Verification items for this drawing (mm, ordinates from the low corner). Coordinates: 2 decimals unless noted, no trailing zeros. Write each loop counter-clockwise with the first axis right and the second up, starting at its lowest first coordinate (ties: lowest second). Pieces come first, ordered by that corner, then holes. Notation, with made-up numbers: (46.5, -0.5) -> (56.5, -0.5) arc R28 ccw to (56.5, 35.5) -> close; hole circle Ø11 at (70.25, 0). An arc over 180 degrees is marked (long way). Answer as CSV lines item,"result".
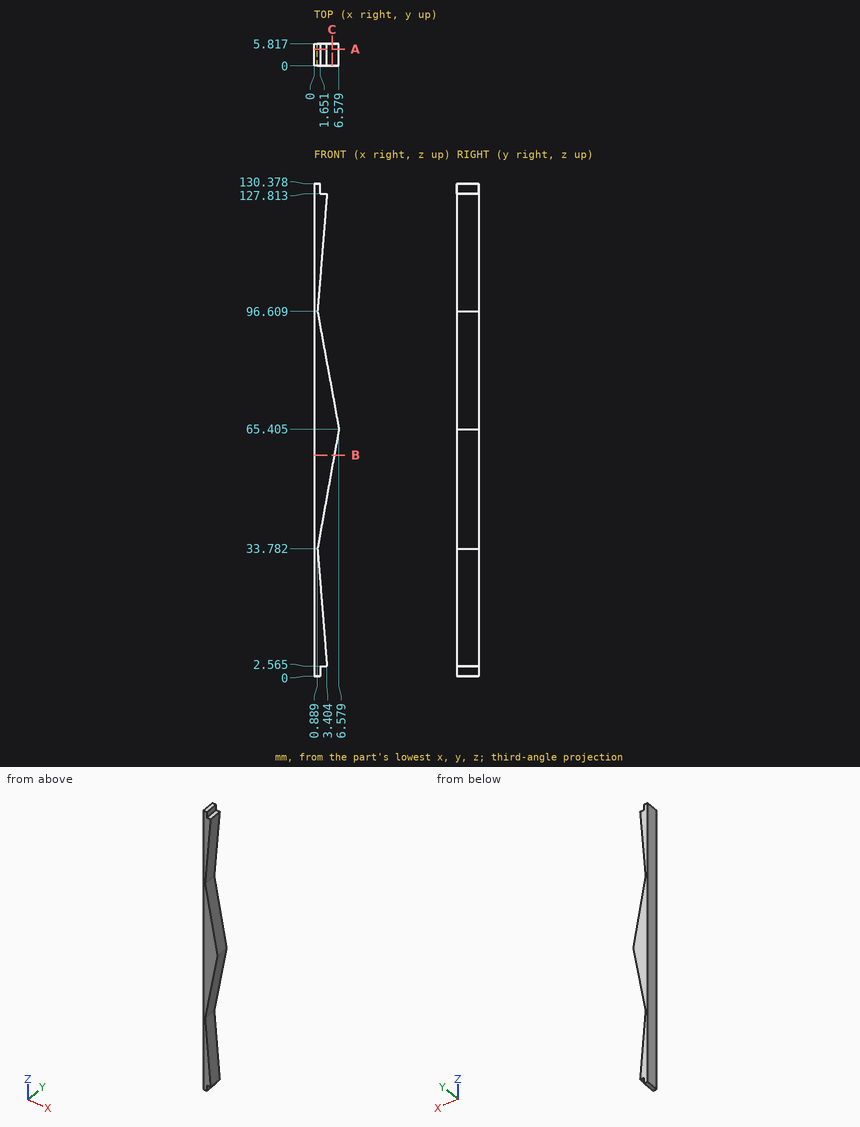
Item 1: Cross-section at B-B, the plane z = 58.5. Record the cut outline in (x, y).
Responses:
outline,"(0, 0) -> (5.34, 0) -> (5.34, 5.82) -> (0, 5.82) -> close"
Item 2: Thickness scan on probe 1 along X at (y, z) = (5.5, 87); probe 2 along X at (y, z) = (1.65, 30.5). Record the ranges inside material, lowest first.
Responses:
probe 1,"x = 0 to 2.64"
probe 2,"x = 0 to 1.15"
Item 3: Depth check by flat-ended pin: pin 1 Ø0.9 at (x, y) = (2.5, 2.5) entering from +Z; pin 2 Ø3 at (y, z) = (1.5, 112) entering from +X; pin 3 Ø0.9 at (x, y) = (2.5, 4.5) entering from -Z (1 decimal). Enter the tip coordinate at first touch or a pass-through.
Responses:
pin 1,"stops at z = 127.81"
pin 2,"stops at x = 2.25"
pin 3,"stops at z = 2.6"
Item 4: Cross-section at C-C, the plane x = 4.75. Record the cut outline in (y, z), plus the area to 3 significant figures.
Responses:
outline,"(0, 55.24) -> (5.82, 55.24) -> (5.82, 75.43) -> (0, 75.43) -> close"
area,"117 mm2"
Item 5: Cross-section at A-A, the plane y = 4.45. Record the cut outline in (x, z) (1 decimal), plus the area to 3 significant figures.
Responses:
outline,"(0, 0) -> (1.7, 0) -> (1.7, 2.6) -> (3.4, 2.6) -> (0.9, 33.8) -> (6.6, 65.4) -> (0.9, 96.6) -> (3.4, 127.8) -> (1.7, 127.8) -> (1.7, 130.4) -> (0, 130.4) -> close"
area,"377 mm2"
